from build123d import *

# Parameters (mm, degrees)
BOSS_EXTRUDE1_DEPTH = 0.1
BOSS_EXTRUDE2_DEPTH = 0.4
BOSS_EXTRUDE3_DEPTH = 1.6
BOSS_EXTRUDE4_DEPTH = 1
BOSS_EXTRUDE6_DEPTH = 2
CUT_EXTRUDE1_DEPTH  = 0.1


with BuildPart() as part:
    # Sketch1 → Boss-Extrude1 (new body)
    with BuildSketch(Plane(origin=(0, 0, 0), x_dir=(1, 0, 0), z_dir=(0, 1, 0))):
        Polygon((-10.646042249, 26.02895066), (-5.401733978, 7.546949539), (-3.551765124, 4.298091631), (5.209504113, 6.784120954), (-1.025832553, 28.758706218), align=None)
    extrude(amount=BOSS_EXTRUDE1_DEPTH)



with BuildPart() as body_2:
    # Sketch1_4 → Boss-Extrude2 (new body)
    with BuildSketch(Plane(origin=(0, 0, 0), x_dir=(1, 0, 0), z_dir=(0, 1, 0))):
        Polygon((11.036175402, 10.498146498), (7.855406085, 33.137420227), (17.758145427, 34.528733828), (20.938914744, 11.889460098), align=None)
    extrude(amount=-BOSS_EXTRUDE2_DEPTH)


with BuildPart() as body_3:
    # Sketch1_6 → Boss-Extrude3 (new body)
    with BuildSketch(Plane(origin=(0, 0, 0), x_dir=(1, 0, 0), z_dir=(0, 1, 0))):
        Polygon((33.147256731, 11.873128664), (34.161951749, 34.390264264), (24.172089788, 34.840439781), (23.15739477, 12.323304181), align=None)
    extrude(amount=-BOSS_EXTRUDE3_DEPTH)


with BuildPart() as body_4:
    # Sketch1_7 → Boss-Extrude4 (new body)
    with BuildSketch(Plane(origin=(0, 0, 0), x_dir=(1, 0, 0), z_dir=(0, 1, 0))):
        Polygon((34.416396618, 6.671846549), (38.325120534, 28.98226014), (48.175095059, 27.256571334), (44.266371143, 4.946157743), align=None)
    extrude(amount=-BOSS_EXTRUDE4_DEPTH)


with BuildPart() as part_1:
    add(part.part)

    add(body_2.part)  # Boss-Extrude6 merges body 2

    add(body_3.part)  # Boss-Extrude6 merges body 3

    add(body_4.part)  # Boss-Extrude6 merges body 4
    # Sketch1_9 → Boss-Extrude6 (add)
    with BuildSketch(Plane(origin=(0, 0, 0), x_dir=(1, 0, 0), z_dir=(0, 1, 0))):
        Polygon((-16.256074113, 26.609004932), (-10.796366677, 29.172241213), (-2.37484271, 31.479114004), (7.84022621, 35.816299809), (16.382403353, 36.668127405), (24.24680656, 37.115536931), (33.214867012, 36.720672561), (36.335094453, 36.39348437), (38.61884098, 31.25680776), (47.446591859, 30.124478905), (52.586728994, 28.662836734), (51.159441766, 18.953851746), (46.768236946, 11.196430212), (45.754807654, 5.085280828), (45.356947793, 0.620078516), (43.361671586, 0.876173274), (23.089608754, 4.521255887), (9.037125491, 1.85322051), (-0.986799702, -0.206421066), align=None)
    extrude(amount=BOSS_EXTRUDE6_DEPTH)

    # Sketch1_11 → Cut-Extrude1 (cut)
    with BuildSketch(Plane(origin=(0, 0, 0), x_dir=(1, 0, 0), z_dir=(0, 1, 0))):
        Polygon((-10.646042249, 26.02895066), (-5.401733978, 7.546949539), (-3.551765124, 4.298091631), (5.209504113, 6.784120954), (-1.025832553, 28.758706218), align=None)
    extrude(amount=CUT_EXTRUDE1_DEPTH, mode=Mode.SUBTRACT)


solid = part_1.part
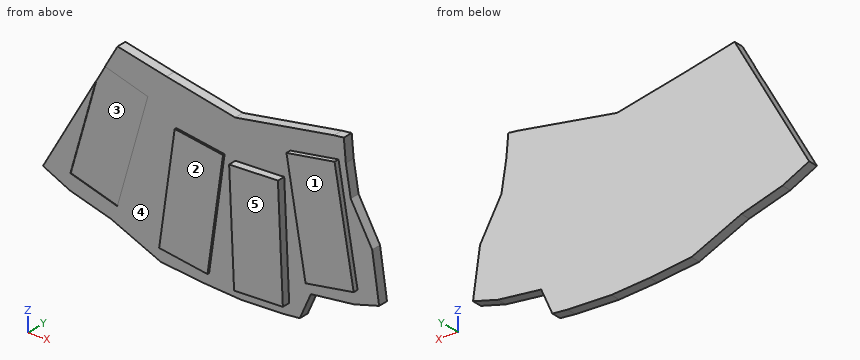
Could you check a few things on this model? Use its own coordinates, in mm. Face numbers are marked on the shaded views. A direction names the side the tool comes from. Coordinates: 2 decimals unless noted, no trailing zeros. Order: outer loops, then holes, each group sorted by start corner. A loop starts at its lowest first (then second) coordinate and runs counter-clockwise, first axis right, second up.
Q1. Suppose I cut it at B-B on z = -25. Please give me the cut outline in (x, y).
Q2. Suppose I cut it at D-D on z = -14.5. Please give me the cut outline in (x, y).
Q3. Which directions (+Z, -Z, +X, -X, +Y, -Y) give clear straight access to the entire face, cutting with the end or side of a thin tool? Please do the marked faces 1, 2 and 3.
Q4. Please list where these lines run through material, in increasing order: L1, parallel to Y at x = 15.5, z = -29; L2, parallel to Y at x = 48, z = -28; L3, parallel to X at y = -0.3, z = -15.5.
Q5. Will these pins go through, and if not, where does the flat tip stop? pin 1 (5 mm diameter, centred on x = -5, z = -22.5, fed in from -Y); pin 2 (4 mm diameter, centred on x = 39.5, z = -19.5, fed in from -Y); pin 3 (5 mm diameter, centred on x = 19.5, z = -12.5, fed in from -Y).
Q6. Thinking about a two-plate mould opening in X: for the marked faces 4 and 5, which applies, released by +X, released by -X, zero draft, split by the parting line, or undercut?
Q7. Suppose I cut it at C-C on x = 40.5. Please give me the cut outline in (y, z).
Q8. Suppose I cut it at A-A on y = 1.25. Please give me the cut outline in (x, z), and give its area (3 significant figures).
Answer:
1. outline: (-15.34, 0) - (-10.35, 0) - (-10.35, 0.1) - (0.04, 0.1) - (0.04, 0) - (9, 0) - (9, -0.4) - (19.1, -0.4) - (19.1, 0) - (23.73, 0) - (23.73, -1.6) - (33.74, -1.6) - (33.74, 0) - (37.63, 0) - (37.63, -1) - (47.78, -1) - (47.78, 0) - (52.05, 0) - (52.05, 2) - (-15.34, 2) - close
2. outline: (-9.36, 0) - (-7.37, 0) - (-7.37, 0.1) - (3.02, 0.1) - (3.02, 0) - (10.47, 0) - (10.47, -0.4) - (20.57, -0.4) - (20.57, 0) - (23.26, 0) - (23.26, -1.6) - (33.27, -1.6) - (33.27, 0) - (35.79, 0) - (35.79, -1) - (45.94, -1) - (45.94, 0) - (48.64, 0) - (48.64, 2) - (-9.36, 2) - close
3. face 1: +Z, -Z, +X, -Y
3. face 2: +Z, -Z, -X, -Y
3. face 3: -Y
4. L1: y = -0.4 to 2
4. L2: y = 0 to 2
4. L3: x = 10.33 to 20.43, 23.3 to 33.31, 35.96 to 46.12
5. pin 1: stops at y = 0.1
5. pin 2: stops at y = -1
5. pin 3: stops at y = -0.4
6. face 4: undercut
6. face 5: zero draft
7. outline: (-1, -28.6) - (0, -28.6) - (0, -31.02) - (2, -31.02) - (2, -1.39) - (0, -1.39) - (0, -5.61) - (-1, -5.61) - close
8. outline: (-16.26, -26.61) - (-10.8, -29.17) - (-2.37, -31.48) - (7.84, -35.82) - (16.38, -36.67) - (24.25, -37.12) - (33.21, -36.72) - (36.34, -36.39) - (38.62, -31.26) - (47.45, -30.12) - (52.59, -28.66) - (51.16, -18.95) - (46.77, -11.2) - (45.75, -5.09) - (45.36, -0.62) - (43.36, -0.88) - (23.09, -4.52) - (9.04, -1.85) - (-0.99, 0.21) - close
8. area: 1,880 mm2
